Work out the finished part from the listing and answer in its coordinate system (mm). A direction names the side the tool comes from. Round coordinates to 2 decimals unless told otherwise and drop trailing zeros. Order: outer loops, then holes, each group sorted by start corner. A loop starts at its lowest first (then second) coordinate and runs counter-clockwise, first axis right, second up. Notation, with made-up numbers: (55.5, 48) - (76.5, 48) arc R31 cw to (76.5, 79) - close; hole circle Ø6 at (-28, 61.5). An arc over 180 degrees is marked (long way). Put each result on its own line as item: value.
```python
from build123d import *

# Parameters (mm, degrees)
F1_DEPTH = 12.7
F2_W     = 50.8
F2_H     = 12.7
F3_DEPTH = 50.8
F4_D     = 25.4
F5_R     = 25.4
F6_R     = 25.39999
F7_R     = 25.4
F8_R     = 25.39999
F10_D    = 25.4


# Not quite as in the source:
# - a fillet or chamfer is up to 0.001 mm smaller than in the source, because OpenCascade refuses the exact size


with BuildPart() as f1:
    # F0 (on Top) → F1 (new body)
    with BuildSketch(Plane.XY):
        with BuildLine():
            ThreePointArc((0, 25.4), (7.4394877579, 7.4394877579), (25.4, 0))
            Line((25.4, 0), (114.3, 0))
            Line((114.3, 0), (114.3, 50.8))
            Line((114.3, 50.8), (25.4, 50.8))
            ThreePointArc((25.4, 50.8), (7.4394877579, 43.3605122421), (0, 25.4))
        make_face()
    extrude(amount=F1_DEPTH)

    # F2 (on face) → F3 (join)
    with BuildSketch(Plane.XY.offset(12.7)):
        with Locations((88.9, 6.35)):
            Rectangle(F2_W, F2_H)
        with Locations((88.9, 44.45)):
            Rectangle(F2_W, F2_H)
    extrude(amount=F3_DEPTH)

    # F4 (through all)
    with Locations(Plane.XY.offset(12.7)):
        with Locations((25.4, 25.4)):
            Hole(F4_D / 2)

    # F5
    f5_edges = [f1.edges().sort_by_distance(p)[0] for p in [
        (63.5, 6.35, 63.5),
    ]]
    fillet(f5_edges, radius=F5_R)

    # F6 (radius 25.4 in the source; OpenCascade refuses exactly that, so slightly less here)
    f6_edges = [f1.edges().sort_by_distance(p)[0] for p in [
        (114.3, 6.35, 63.5),
    ]]
    fillet(f6_edges, radius=F6_R)

    # F7
    f7_edges = [f1.edges().sort_by_distance(p)[0] for p in [
        (63.5, 44.45, 63.5),
    ]]
    fillet(f7_edges, radius=F7_R)

    # F8 (radius 25.4 in the source; OpenCascade refuses exactly that, so slightly less here)
    f8_edges = [f1.edges().sort_by_distance(p)[0] for p in [
        (114.3, 44.45, 63.5),
    ]]
    fillet(f8_edges, radius=F8_R)

    # F10 (through all)
    with Locations(Plane.XZ):
        with Locations((88.9, 38.1)):
            Hole(F10_D / 2)


solid = f1.part
```
1) For a pull along X with two mould halves and no side action, classify faces 4 (the cylindrical face through (70.74, 6.44, 55.86)), 5 (the cylindrical face through (106.66, 6.44, 56.26)), 6 (the cylindrical face through (18.573, 36.109, 6.261)) as pulls with the +X half, pulls with the -X half, needs draft (parallel to the pull), parting line crosses it, or undercut.
Findings below:
face 4: pulls with the -X half
face 5: pulls with the +X half
face 6: undercut
2) A cutting plane is placed at B-B on z = 20. Write down the section's boundary in (x, y).
Findings below:
outline: (63.5, 0) - (114.3, 0) - (114.3, 12.7) - (63.5, 12.7) - close; (63.5, 38.1) - (114.3, 38.1) - (114.3, 50.8) - (63.5, 50.8) - close
3) For faces 1 (the flat face through (79, 0, 24)), 2 (the flat face through (83, 12.7, 26)), 3 (the flat face through (63.5, 44, 25)), determine the directions among +Z, -Z, +X, -X, +Y, -Y from which every point of the face is accessible in a straight line to the end or side of a thin tool.
Findings below:
face 1: +Z, -Z, +X, -X, -Y
face 2: +Z, +X, -X
face 3: +Z, -X, +Y, -Y
4) Straight lines are drawn through the part: L1, parallel to Y at x = 82, z = 26.5; L2, parallel to X at y = 4, z = 38; L3, parallel to Z at x = 69, y = 15.5. For each, find the intervals that lie inside material, in ascending order. Write a range as from..to.
Findings below:
L1: y = 0..12.7, 38.1..50.8
L2: x = 63.5..76.2, 101.6..114.3
L3: z = 0..12.7
5) Given pin 1 Ø8 at (x, y) = (56, 16.5) entering from -Z; pin 2 Ø8 at (x, y) = (53.5, 42.5) entering from +Z; pin 3 Ø10 at (y, z) = (6.5, 28.5) entering from -X; pin 4 Ø4 at (y, z) = (11, 42.5) entering from +X, each flat-ended and moving along its own axis, determine where each tip first touches the part or whether it passes through.
Findings below:
pin 1: stops at z = 0
pin 2: stops at z = 12.7
pin 3: stops at x = 63.5
pin 4: stops at x = 114.19
6) A cutting plane is placed at C-C on x = 16. Write down the section's boundary in (y, z), then the cut area to 3 significant figures.
Findings below:
outline: (1.8, 0) - (16.86, 0) - (16.86, 12.7) - (1.8, 12.7) - close; (33.94, 0) - (49, 0) - (49, 12.7) - (33.94, 12.7) - close
area: 382 mm2
7) A cutting plane is placed at A-A on x = 81. Write down the section's boundary in (y, z).
Findings below:
outline: (0, 0) - (50.8, 0) - (50.8, 28.16) - (38.1, 28.16) - (38.1, 12.7) - (12.7, 12.7) - (12.7, 28.16) - (0, 28.16) - close; (0, 48.04) - (12.7, 48.04) - (12.7, 62.24) - (0, 62.24) - close; (38.1, 48.04) - (50.8, 48.04) - (50.8, 62.24) - (38.1, 62.24) - close
